The model under review builds one solid part; all positions refer to its coordinate system, in mm. Give positions to 0.01 mm unless a question says otherwise; leave off trailing zeros. Order: outer loops, then holes, each group sorted by start corner. A loop starts at its lowest first (then second) coordinate and runs counter-clockwise, first axis right, second up.
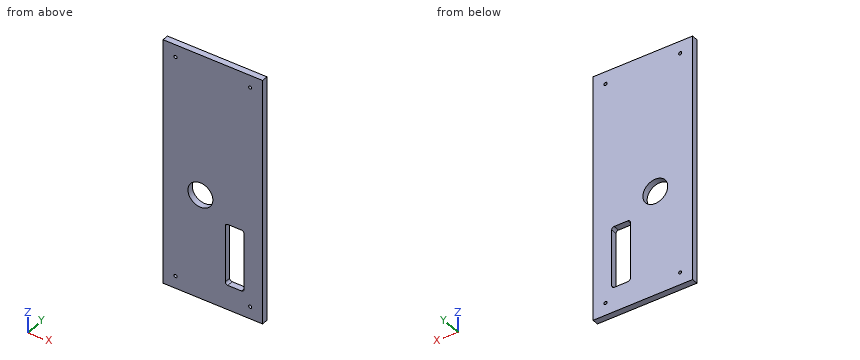
```python
from build123d import *

# Parameters (mm, degrees)
SKETCH1_W           = 101.6
SKETCH1_H           = 254
SKETCH1_R           = 12.7
SKETCH1_R_2         = 1.5875
BOSS_EXTRUDE1_DEPTH = 6.35


with BuildPart() as part:
    # Sketch1 → Boss-Extrude1 (new body)
    with BuildSketch(Plane(origin=(0, 0, 0), x_dir=(1, 0, 0), z_dir=(0, 1, 0))):
        Rectangle(SKETCH1_W, SKETCH1_H)
        with Locations((-12.7, 19.05)):
            Circle(SKETCH1_R, mode=Mode.SUBTRACT)
        with Locations((-38.1, -114.3)):
            Circle(SKETCH1_R_2, mode=Mode.SUBTRACT)
        with Locations((38.1, -114.3)):
            Circle(SKETCH1_R_2, mode=Mode.SUBTRACT)
        with Locations((38.1, 114.3)):
            Circle(SKETCH1_R_2, mode=Mode.SUBTRACT)
        with Locations((-38.1, 114.3)):
            Circle(SKETCH1_R_2, mode=Mode.SUBTRACT)
        with BuildLine():
            Line((29.21, 101.6), (15.24, 101.6))
            ThreePointArc((15.24, 101.6), (13.443948776, 100.856051224), (12.7, 99.06))
            Line((12.7, 99.06), (12.7, 40.64))
            ThreePointArc((12.7, 40.64), (13.443948776, 38.843948776), (15.24, 38.1))
            Line((15.24, 38.1), (29.21, 38.1))
            ThreePointArc((29.21, 38.1), (31.006051224, 38.843948776), (31.75, 40.64))
            Line((31.75, 40.64), (31.75, 99.06))
            ThreePointArc((31.75, 99.06), (31.006051224, 100.856051224), (29.21, 101.6))
        make_face(mode=Mode.SUBTRACT)
    extrude(amount=BOSS_EXTRUDE1_DEPTH)


solid = part.part
```
1. Take a section at B-B (y = 2.75). Count the separate pieces of the cut face and the enclosed holes in it, and give its area (3 significant figures).
2. Insertion check: pin 1 (1.9 mm diameter, centred on x = 38.1, z = -114.3, fed in from -Y). The pin has a flat end and moves straight along its axis. Give the tip position at first contact, or say it passes through.
3. Take a section at A-A (z = -71.5). Write out the cut boundary in (x, y).
4. Take a section at C-C (x = -12.7). Write out the cut boundary in (y, z), and give its area (3 significant figures).
5. To check wall thickness, follow line 1 (Z direction, x = -38.1, y = 3.25); line 2 (X direction, y = 1.5, z = 114.3); line 3 (X direction, y = 3, z = -93). State the ranges of each line that lie inside material, in increasing order.
Answer:
1. separate pieces: 1
1. enclosed holes: 6
1. area: 24,100 mm2
2. pin 1: passes through
3. outline: (-50.8, 0) - (12.7, 0) - (12.7, 6.35) - (-50.8, 6.35) - close; (31.75, 0) - (50.8, 0) - (50.8, 6.35) - (31.75, 6.35) - close
4. outline: (0, -127) - (6.35, -127) - (6.35, -31.75) - (0, -31.75) - close; (0, -6.35) - (6.35, -6.35) - (6.35, 127) - (0, 127) - close
4. area: 1,450 mm2
5. line 1: z = -127 to -115.89, -112.71 to 112.71, 115.89 to 127
5. line 2: x = -50.8 to -39.69, -36.51 to 36.51, 39.69 to 50.8
5. line 3: x = -50.8 to 12.7, 31.75 to 50.8
